Source: three-view drawing plus pictorial views. Frame: mm from the lowest corner of the part. A direction names the side the tool comes from. Give positions to 0.01 mm unless a question says otherwise; leave off trailing zeros. Loops run counter-clockwise (first coordinate to the right, second up) from the corner with the lowest first, then second, coordinate; pieces in that order, holes last. Notation, with made-up numbers: M 60,-0.5 L 117,-0.5 A31 ccw 117,29.5 Z; hole C 9.5,-24.5 d10. An arc over 180 degrees is marked long. Write item = value, one per line.
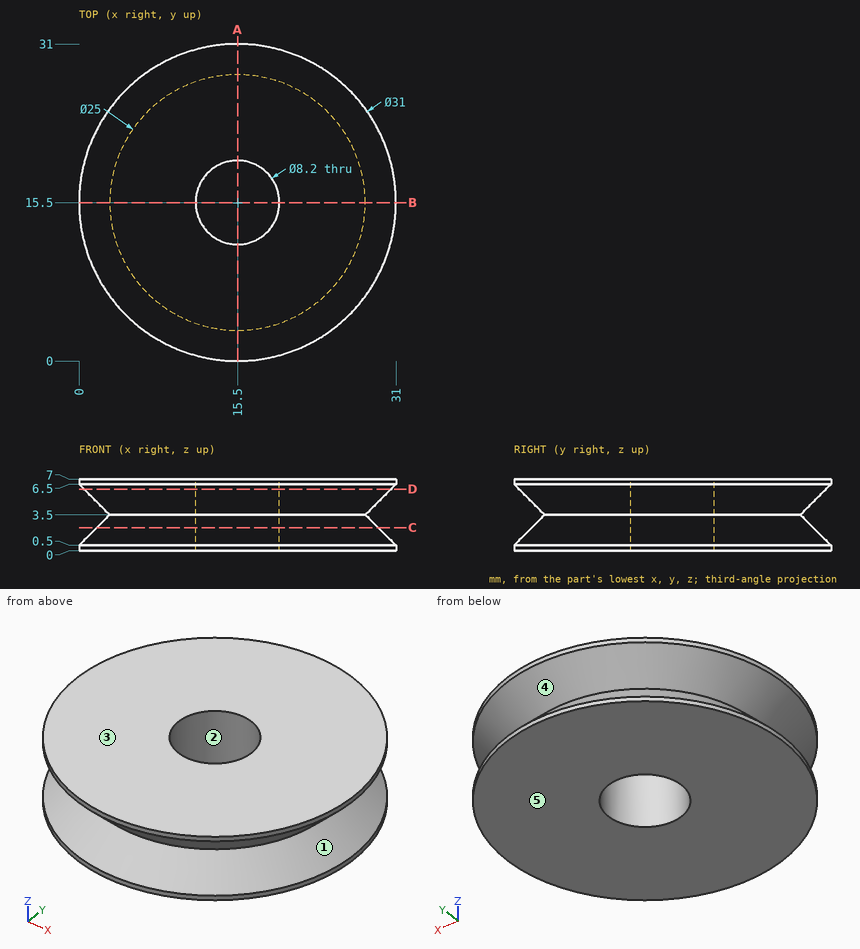
1. Cut plane C-C, the plane z = 2.25. Return the cut outline in (x, y).
Derived:
outline = C 15.5,15.5 d27.5; hole C 15.5,15.5 d8.2
2. Cut plane A-A, the plane x = 15.5. Return the cut outline in (y, z).
Derived:
outline = M 0,0 L 11.4,0 L 11.4,7 L 0,7 L 0,6.5 L 3,3.5 L 0,0.5 Z; M 19.6,0 L 31,0 L 31,0.5 L 28,3.5 L 31,6.5 L 31,7 L 19.6,7 Z
3. Cut plane D-D, the plane z = 6. Return the cut outline in (x, y), then the cut area to 3 significant figures.
Derived:
outline = C 15.5,15.5 d30; hole C 15.5,15.5 d8.2
area = 654 mm²
4. First-contact query: pin 1 Ø4 at (y, z) = (5, 4.5) entering from +X; pin 2 Ø1 at (y, z) = (22.5, 2.5) entering from -X; pin 3 Ø2 at (x, z) = (10.5, 3) entering from +Y. Flat tips, straight axial feed; report the tip coordinate or a pass-through.
Derived:
pin_1 = 27.41
pin_2 = 3.31
pin_3 = 28.64
5. Pull-direction query (X, two-part tool) for the marked faces 1, 2 and 3; classes: +X half, -X half, draft (parallel to the pull), parting line (faces both ways), or undercut.
Derived:
face_1 = parting line
face_2 = undercut
face_3 = draft
6. Material intervals for probe 1 along X at (y, z) = (17.5, 2); probe 2 along Y at (x, z) = (13.5, 4); probe 3 along Y at (x, z) = (15.5, 4.5), sorted ascending. Write a range as from..to.
Derived:
probe_1 = 1.64..11.92, 19.08..29.36
probe_2 = 2.65..11.92, 19.08..28.35
probe_3 = 2..11.4, 19.6..29
7. Reachability of the marked faces 4 and 5 from +Z, -Z, +X, -X, +Y, -Y: full face, straight path, thin tool, end or side. Return the list, or none.
Derived:
face_4 = none
face_5 = -Z, +X, -X, +Y, -Y
